from build123d import *

# Parameters (mm, degrees)
BOSS_EXTRUDE1_DEPTH = 1
SKETCH4_W           = 0.5
SKETCH4_H           = 5
BOSS_EXTRUDE2_DEPTH = 0.15


with BuildPart() as part:
    # Sketch1 → Revolve1 (revolve)
    with BuildSketch(Plane.XY):
        with BuildLine():
            Line((2.5, 4.02324589), (2.5, -1.07675411))
            Line((2.5, -1.07675411), (0, -1.07675411))
            Line((0, -1.07675411), (0, 6.52324589))
            ThreePointArc((0, 6.52324589), (1.767766953, 5.791012843), (2.5, 4.02324589))
        make_face()
    revolve(axis=Axis((0, -170.01390881, 0), (0, 1, 0)))

    # Sketch2 → Boss-Extrude1 (add)
    with BuildSketch(Plane.XZ.offset(1.07675411)):
        with BuildLine():
            Line((2.10585574, -2.065882766), (2.777744802, 0.993294426))
            ThreePointArc((2.777744802, 0.993294426), (-2.88132432, 0.632827121), (2.10585574, -2.065882766))
        make_face()
    extrude(amount=BOSS_EXTRUDE1_DEPTH)

    # Sketch4 → Boss-Extrude2 (add, symmetric)
    with BuildSketch(Plane.XY):
        with Locations((1.52, -4.57675411)):
            Rectangle(SKETCH4_W, SKETCH4_H)
        with Locations((-1.52, -4.57675411)):
            Rectangle(SKETCH4_W, SKETCH4_H)
    extrude(amount=BOSS_EXTRUDE2_DEPTH, both=True)


solid = part.part
The model under review builds one solid part; all positions refer to its coordinate system, in mm. A direction names the side the tool comes from. Give positions to 0.01 mm unless a question says otherwise; leave off trailing zeros. Order: outer loops, then holes, each group sorted by start corner. A loop starts at its lowest first (then second) coordinate and runs counter-clockwise, first axis right, second up. Notation, with made-up numbers: (60.5, -7) -> (99.5, -7) arc R29 cw to (99.5, 27) -> close; hole circle Ø4 at (1, 27.25). An arc over 180 degrees is marked (long way). Write item = value, one per line. Start each with the question number.
(1) For pin 1 Ø1.5 at (y, z) = (2.5, 1.5) entering from +X; pin 2 Ø1 at (y, z) = (2, -1) entering from -X; pin 3 Ø3 at (y, z) = (-2, -0.5) entering from -X; pin 4 Ø0.6 at (x, y) = (-1.5, -5.5) entering from +Z, all flat-tipped, find the tip position at first contact; note any pin that passes through.
(2) Take a section at A-A (y = -2.25). Write out the cut boundary in (x, z), plus the area to 3 significant figures.
(3) Take a section at D-D (y = 2.5). Write out the cut boundary in (x, z).
(4) Tool access review of faces 1 (the cylindrical face through (-2.857, -1.57, 0.737)), 2 (the cylindrical face through (-0.54, 1.44, 2.44)): name each direction out of +Z, -Z, +X, -X, +Y, -Y from which nothing blocks a thin tool from reaching the whole face with its end or side.
(5) For L1, parallel to X at y = -5.5, z = -0.05; L2, parallel to Y at x = -2.5, z = 0.8; L3, parallel to Z at x = 0, y = 1.75, list the stretches that pass through material, from the lowest coordinate up. Write a range as from..to.
(6) Take a section at B-B (x = 0). Write out the cut boundary in (y, z), plus the area to 3 significant figures.
Returned:
q1.pin_1 = 2.38
q1.pin_2 = -2.45
q1.pin_3 = -2.95
q1.pin_4 = 0.15
q2.outline = (-1.77, -0.15) -> (-1.27, -0.15) -> (-1.27, 0.15) -> (-1.77, 0.15) -> close; (1.27, -0.15) -> (1.77, -0.15) -> (1.77, 0.15) -> (1.27, 0.15) -> close
q2.area = 0.300 mm²
q3.outline = circle Ø5 at (0, 0)
q4.face_1 = +Y, -Y
q4.face_2 = +Y
q5.L1 = -1.77..-1.27, 1.27..1.77
q5.L2 = -2.08..-1.08
q5.L3 = -2.5..2.5
q6.outline = (-2.08, -2.95) -> (-1.08, -2.95) -> (-1.08, -2.5) -> (4.02, -2.5) arc R2.5 ccw to (4.02, 2.5) -> (-1.08, 2.5) -> (-1.08, 2.95) -> (-2.08, 2.95) -> close
q6.area = 41.2 mm²
